from build123d import *

# Parameters (mm, degrees)
SKETCH_1_W          = 20
SKETCH_1_H          = 20
EXTRUDE_1_DEPTH     = 100
CUT_EXTRUDE_1_DEPTH = 34
CUT_EXTRUDE_2_DEPTH = 34
CUT_EXTRUDE_3_DEPTH = 34


with BuildPart() as part:
    # 草图1 → 凸台-拉伸1 (new body)
    with BuildSketch(Plane(origin=(0, 0, 0), x_dir=(0, 0, -1), z_dir=(1, 0, 0))):
        Rectangle(SKETCH_1_W, SKETCH_1_H)
    extrude(amount=EXTRUDE_1_DEPTH)

    # 草图2 → 切除-拉伸1 (cut)
    with BuildSketch(Plane.XY.offset(10)):
        Polygon((100, 10), (90, 10), (100, 0), align=None)
    extrude(amount=-CUT_EXTRUDE_1_DEPTH, mode=Mode.SUBTRACT)

    # 草图3 → 切除-拉伸2 (cut)
    with BuildSketch(Plane.XY.offset(10)):
        Polygon((100, 0), (100, -10), (90, -10), align=None)
    extrude(amount=-CUT_EXTRUDE_2_DEPTH, mode=Mode.SUBTRACT)

    # 草图4 → 切除-拉伸3 (cut)
    with BuildSketch(Plane(origin=(0, 10, 0), x_dir=(1, 0, 0), z_dir=(0, 1, 0))):
        Polygon((100, 10), (90, 10), (100, 0), align=None)
        Polygon((90, -10), (100, -10), (100, 0), align=None)
    extrude(amount=-CUT_EXTRUDE_3_DEPTH, mode=Mode.SUBTRACT)


solid = part.part
Check sheet for the modelled part. Datum: model origin and axes. Units: mm. Coordinates: 2 decimals unless noted, no trailing zeros. Loops run counter-clockwise (first coordinate to the right, second up) from the corner with the lowest first, then second, coordinate; pieces in that order, holes last. Notation, with made-up numbers: (10.25, 56) -> (25.25, 56) arc R23 ccw to (25.25, 80) -> close; hole circle Ø10 at (-0.5, -1.75). An arc over 180 degrees is marked (long way). Write item = value, one per line. Start each with the question number.
1. Material ranges on line 1 (X direction, y = 2.5, z = -8.75); line 2 (X direction, y = -3.75, z = 9); line 3 (Z direction, x = 96, y = -2), recorded low to high.
2. Section check B-B on y = 6. Record the cut outline in (x, z), then the cut area to 3 significant figures.
3. Section check A-A on z = 7.25. Record the cut outline in (x, y).
4. Depth check by flat-ended pin: P1, Ø12, axis at y = -4.5, z = 6, coming from the -X side; P2, Ø10, axis at y = -4, z = -5, coming from the +X side; P3, Ø1, axis at y = 7, z = 7.5, coming from the +X side; P4, Ø1.5, axis at y = -6, z = -4.5, coming from the +X side. Enter the tip coordinate at first touch or a pass-through.
Responses:
q1.line_1 = 0 to 91.25
q1.line_2 = 0 to 91
q1.line_3 = -4 to 4
q2.outline = (0, -10) -> (90, -10) -> (94, -6) -> (94, 6) -> (90, 10) -> (0, 10) -> close
q2.area = 1,860 mm2
q3.outline = (0, -10) -> (90, -10) -> (92.75, -7.25) -> (92.75, 7.25) -> (90, 10) -> (0, 10) -> close
q4.P1 = 0
q4.P2 = 99
q4.P3 = 93
q4.P4 = 94.75
